from build123d import *

# Parameters (mm, degrees)
SKETCH1_R           = 42.5
SKETCH1_R_2         = 40
BOSS_EXTRUDE1_DEPTH = 10
BOSS_EXTRUDE2_START = -5
BOSS_EXTRUDE2_DEPTH = 5
SKETCH3_R           = 4
SKETCH3_R_2         = 3
BOSS_EXTRUDE3_DEPTH = 2
SKETCH4_R           = 3
CUT_EXTRUDE1_DEPTH  = 64.344297297
BOSS_EXTRUDE4_START = 15
BOSS_EXTRUDE4_DEPTH = 15


with BuildPart() as part:
    # Sketch1 → Boss-Extrude1 (new, symmetric)
    with BuildSketch(Plane(origin=(0, 0, 0), x_dir=(1, 0, 0), z_dir=(0, 1, 0))):
        with Locations(Location((0, 0, 0), (0, 0, 270))):
            Circle(SKETCH1_R)
        with Locations(Location((0, 0, 0), (0, 0, 270))):
            Circle(SKETCH1_R_2, mode=Mode.SUBTRACT)
    extrude(amount=BOSS_EXTRUDE1_DEPTH, both=True)

    # Sketch2 → Boss-Extrude2 (add)
    with BuildSketch(Plane(origin=(0, 10, 0), x_dir=(1, 0, 0), z_dir=(0, 1, 0)).offset(BOSS_EXTRUDE2_START)):
        with BuildLine():
            ThreePointArc((-38.889408297, 9.36023089), (-14.142135624, 14.142135624), (-9.36023089, 38.889408297))
            ThreePointArc((-9.36023089, 38.889408297), (0, 40), (9.36023089, 38.889408297))
            ThreePointArc((9.36023089, 38.889408297), (14.142135624, 14.142135624), (38.889408297, 9.36023089))
            ThreePointArc((38.889408297, 9.36023089), (40, 0), (38.889408297, -9.36023089))
            ThreePointArc((38.889408297, -9.36023089), (14.142135624, -14.142135624), (9.36023089, -38.889408297))
            ThreePointArc((9.36023089, -38.889408297), (0, -40), (-9.36023089, -38.889408297))
            ThreePointArc((-9.36023089, -38.889408297), (-14.142135624, -14.142135624), (-38.889408297, -9.36023089))
            ThreePointArc((-38.889408297, -9.36023089), (-40, 0), (-38.889408297, 9.36023089))
        make_face()
    extrude(amount=BOSS_EXTRUDE2_DEPTH)

    # Sketch3 → Boss-Extrude3 (add)
    with BuildSketch(Plane(origin=(0, 10, 0), x_dir=(1, 0, 0), z_dir=(0, 1, 0))):
        with Locations(Location((0, 0, 0), (0, 0, 270))):
            Circle(SKETCH3_R)
        with Locations(Location((0, 0, 0), (0, 0, 270))):
            Circle(SKETCH3_R_2, mode=Mode.SUBTRACT)
    extrude(amount=BOSS_EXTRUDE3_DEPTH)

    # Sketch4 → Cut-Extrude1 (cut, through all)
    with BuildSketch(Plane(origin=(0, 10, 0), x_dir=(1, 0, 0), z_dir=(0, 1, 0))):
        with Locations(Location((0, 0, 0), (0, 0, 270))):
            Circle(SKETCH4_R)
    extrude(amount=-CUT_EXTRUDE1_DEPTH, mode=Mode.SUBTRACT)

    # Sketch5 → Boss-Extrude4 (add)
    with BuildSketch(Plane.XZ.offset(-5).offset(BOSS_EXTRUDE4_START)):
        with BuildLine():
            Line((-25, -8.126552801), (-25, 8.126552801))
            ThreePointArc((-25, 8.126552801), (-32.042685029, 7.64027064), (-38.889408297, 9.36023089))
            ThreePointArc((-38.889408297, 9.36023089), (-40, 0), (-38.889408297, -9.36023089))
            ThreePointArc((-38.889408297, -9.36023089), (-32.042685029, -7.64027064), (-25, -8.126552801))
        make_face()
        with BuildLine():
            Line((-8.126552801, 25), (8.126552801, 25))
            ThreePointArc((8.126552801, 25), (7.64027064, 32.042685029), (9.36023089, 38.889408297))
            ThreePointArc((9.36023089, 38.889408297), (0, 40), (-9.36023089, 38.889408297))
            ThreePointArc((-9.36023089, 38.889408297), (-7.64027064, 32.042685029), (-8.126552801, 25))
        make_face()
        with BuildLine():
            Line((25, 8.126552801), (25, -8.126552801))
            ThreePointArc((25, -8.126552801), (32.042685029, -7.64027064), (38.889408297, -9.36023089))
            ThreePointArc((38.889408297, -9.36023089), (40, 0), (38.889408297, 9.36023089))
            ThreePointArc((38.889408297, 9.36023089), (32.042685029, 7.64027064), (25, 8.126552801))
        make_face()
        with BuildLine():
            Line((8.126552801, -25), (-8.126552801, -25))
            ThreePointArc((-8.126552801, -25), (-7.64027064, -32.042685029), (-9.36023089, -38.889408297))
            ThreePointArc((-9.36023089, -38.889408297), (0, -40), (9.36023089, -38.889408297))
            ThreePointArc((9.36023089, -38.889408297), (7.64027064, -32.042685029), (8.126552801, -25))
        make_face()
    extrude(amount=-BOSS_EXTRUDE4_DEPTH)


solid = part.part
Geometry: final body of the model. Coordinates: model frame, mm. A direction names the side the tool comes from. Coordinates: 2 decimals unless noted, no trailing zeros. Order: outer loops, then holes, each group sorted by start corner. A loop starts at its lowest first (then second) coordinate and runs counter-clockwise, first axis right, second up.
1) Ray query, probe 1 along X at (y, z) = (-5, -33); probe 2 along X at (y, z) = (-6.5, -34); probe 3 along Z at (x, y) = (-32, -5.25). Return the intervals inside material, ascending.
Result sheet:
probe 1: x = -26.78 to -22.61, -7.75 to 7.75, 22.61 to 26.78
probe 2: x = -25.5 to -21.07, -7.9 to 7.9, 21.07 to 25.5
probe 3: z = -27.97 to -24, -7.64 to 7.64, 24 to 27.97
2) First-contact query: P1, Ø4, axis at y = 3, z = -10, coming from the -X side; P2, Ø8, axis at x = -15, z = 20, coming from the +Y side; P3, Ø9.5, axis at x = 0, z = 0, coming from the -Y side; P4, Ø1, axis at x = 5.5, y = -2.5, coming from the -Z side. Flat tips, straight axial feed; report the tip coordinate or a pass-through.
Result sheet:
P1: stops at x = -41.74
P2: passes through
P3: stops at y = 5
P4: stops at z = -42.2
3) Section D-D (z = 0). Return loops of the section in (x, y), then the cut area to 3 significant figures.
Result sheet:
outline: (-42.5, -10) - (-25, -10) - (-25, 5) - (-3, 5) - (-3, 12) - (-4, 12) - (-4, 10) - (-42.5, 10) - close; (3, 5) - (25, 5) - (25, -10) - (42.5, -10) - (42.5, 10) - (4, 10) - (4, 12) - (3, 12) - close
area: 924 mm2
4) Section A-A (y = 7.5). Return loops of the section in (x, z), then the cut area to 3 significant figures.
Result sheet:
outline: circle Ø85 at (0, 0); hole (-38.89, -9.36) arc R40 ccw to (-9.36, -38.89) arc R22.5 ccw to start; hole (-38.89, 9.36) arc R22.5 ccw to (-9.36, 38.89) arc R40 ccw to start; hole circle Ø6 at (0, 0); hole (9.36, -38.89) arc R40 ccw to (38.89, -9.36) arc R22.5 ccw to start; hole (9.36, 38.89) arc R22.5 ccw to (38.89, 9.36) arc R40 ccw to start
area: 3,270 mm2
5) Draft query along X for faces 1 (the cylindrical face through (-3.905, 10.986, -0.867)), 2 (the flat face through (-25, -3, 0)), 3 (the flat face through (3, 12, 1)). Return one class per face: released by +X, released by -X, zero draft, split by the parting line, or undercut.
Result sheet:
face 1: split by the parting line
face 2: undercut
face 3: zero draft
6) Set-up query: faces 4 (the flat face through (-25.4, -10, 0.2)), 5 (the cylindrical face through (-28.066, -0.14, -28.501)), 6 (the flat face through (6, 5, 0)). Return all of +Z, -Z, +X, -X, +Y, -Y with unobstructed straight access to the full face (end or side cutting, diameter ignored); none if empty.
Result sheet:
face 4: +Z, -Z, +X, -X, -Y
face 5: +Y, -Y
face 6: -Y
7) Section C-C (y = -4.5). Return loops of the section in (x, z), then the cut area to 3 significant figures.
Result sheet:
outline: circle Ø85 at (0, 0); hole (-38.89, -9.36) arc R40 ccw to (-9.36, -38.89) arc R22.5 ccw to (-8.13, -25) - (8.13, -25) arc R22.5 ccw to (9.36, -38.89) arc R40 ccw to (38.89, -9.36) arc R22.5 ccw to (25, -8.13) - (25, 8.13) arc R22.5 ccw to (38.89, 9.36) arc R40 ccw to (9.36, 38.89) arc R22.5 ccw to (8.13, 25) - (-8.13, 25) arc R22.5 ccw to (-9.36, 38.89) arc R40 ccw to (-38.89, 9.36) arc R22.5 ccw to (-25, 8.13) - (-25, -8.13) arc R22.5 ccw to start
area: 1,590 mm2
8) Section B-B (x = 0). Return loops of the section in (y, z).
Result sheet:
outline: (-10, -42.5) - (10, -42.5) - (10, -4) - (12, -4) - (12, -3) - (5, -3) - (5, -25) - (-10, -25) - close; (-10, 25) - (5, 25) - (5, 3) - (12, 3) - (12, 4) - (10, 4) - (10, 42.5) - (-10, 42.5) - close
